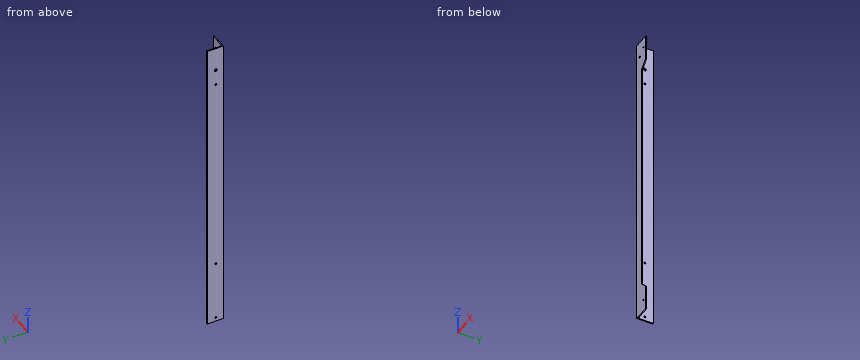
Autodesk Inventor part; units mm, degrees
ref_plane "YZ Plane" through (0, 0, 0) normal (1, 0, 0) x (0, 1, 0)
ref_plane "XZ Plane" through (0, 0, 0) normal (0, 1, 0) x (-1, 0, 0)
ref_plane "XY Plane" through (0, 0, 0) normal (0, 0, 1) x (1, 0, 0)
sketch "Sketch1" plane through (0, 0, 0) normal (0, 0, 1) x (1, 0, 0)
  line L0 (0, 0) -> (3.175, 0)
  line L1 (3.175, 0) -> (3.175, 50.8)
  line L2 (3.175, 50.8) -> (0, 50.8)
  line L3 (0, 50.8) -> (0, 0)
  line L4 (0, 0) -> (50.8, 0)
  line L5 (50.8, 0) -> (50.8, 3.175)
  line L6 (50.8, 3.175) -> (0, 3.175)
  line L7 (0, 3.175) -> (0, 0)
  dimension "d0" = 3.175
  dimension "d1" = 50.8
  dimension "d2" = 50.8
  dimension "d3" = 3.175
extrude "Extrusion1" add sketch "Sketch1" along normal blind 965.2
sketch "Sketch2" plane through (0, 0, 0) normal (-1, 0, 0) x (0, 0, 1)
  line L0 (0, 50.8) -> (0, 0)
  line L1 (0, 0) -> (965.2, 0)
  point P0 (12.7, 23.8125)
  point P1 (203.2, 23.8125)
  dimension "d6" = 23.8125
  dimension "d7" = 23.8125
  dimension "d8" = 12.7
  dimension "d9" = 203.2
hole "Hole1" at (0, 23.8125, 12.7) at (0, 23.8125, 203.2) direction (1, 0, 0) diameter 6.35 end through all
sketch "Sketch3" plane through (0, 0, 0) normal (-1, 0, 0) x (0, 0, 1)
  line L0 (0, 0) -> (965.2, 0)
  line L1 (0, 50.8) -> (0, 0)
  point P0 (889, 23.8125)
  dimension "d17" = 23.8125
  dimension "d26" = 889
hole "Hole2" at (0, 23.8125, 889) direction (1, 0, 0) diameter 9.525 end through all
sketch "Sketch4" plane through (0, 0, 0) normal (0, -1, 0) x (1, 0, 0)
  line L0 (0, 965.2) -> (50.8, 965.2)
  line L1 (0, 0) -> (0, 965.2)
  point P0 (17.4625, 914.4)
  dimension "d27" = 17.4625
  dimension "d28" = 50.8
hole "Hole3" at (17.4625, 0, 914.4) direction (0, 1, 0) diameter 6.35 end through all
fillet "Fillet1" radius 3.175 1 edges at (3.175, 3.175, 482.6)
sketch "Sketch6" plane through (0, 0, 0) normal (0, -1, 0) x (1, 0, 0)
  line L0 (0, 0) -> (50.8, 0)
  line L1 (50.8, 0) -> (50.8, 965.2)
  line L2 (0, 965.2) -> (50.8, 965.2)
  point P0 (38.1, 933.45)
  point P1 (38.1, 38.1)
  dimension "d49" = 38.1
  dimension "d50" = 12.7
  dimension "d51" = 31.75
  dimension "d52" = 12.7
hole "Hole5" at (38.1, 0, 933.45) at (38.1, 0, 38.1) direction (0, 1, 0) diameter 4.7625 end through all
sketch "Sketch8" plane through (0, 0, 0) normal (0, -1, 0) x (1, 0, 0)
  circle A0 centre (38.1, 933.45) radius 2.3813
  circle A1 centre (38.1, 38.1) radius 2.3813
  circle A2 centre (17.4625, 914.4) radius 3.175
  line L0 (0, 0) -> (50.8, 0)
  line L1 (50.8, 0) -> (50.8, 965.2)
  line L2 (0, 965.2) -> (50.8, 965.2)
  line L3 (0, 0) -> (0, 965.2)
  line L4 (50.8, 863.6) -> (28.575, 863.6)
  line L5 (28.575, 863.6) -> (28.575, 101.6)
  line L6 (28.575, 101.6) -> (50.8, 101.6)
  line L7 (50.8, 101.6) -> (50.8, 863.6)
  line L8 (28.575, 863.6) -> (50.8, 885.825)
  line L9 (50.8, 0) -> (50.8, 965.2)
  line L10 (28.575, 863.6) -> (60.0059, 863.6) construction
  line L11 (50.8, 885.825) -> (50.8, 863.6)
  line L12 (28.575, 101.6) -> (50.8, 79.375)
  line L13 (28.575, 101.6) -> (60.0059, 101.6) construction
  line L14 (50.8, 79.375) -> (50.8, 101.6)
  dimension "d60" = 22.225
  dimension "d61" = 101.6
  dimension "d62" = 101.6
  dimension "d63" = 45
  dimension "d64" = 45
extrude "Extrusion2" cut sketch "Sketch8" against normal blind 25.4 contours L12 L6 L1 | L6 L5 L4 L1 | L1 L4 L8
sketch "Sketch9" plane through (0, 0, 0) normal (-1, 0, 0) x (0, 0, 1)
  circle A0 centre (889, 23.8125) radius 4.7625
  circle A1 centre (12.7, 23.8125) radius 3.175
  circle A2 centre (203.2, 23.8125) radius 3.175
  line L0 (0, 50.8) -> (0, 0)
  line L1 (0, 0) -> (965.2, 0)
  line L2 (965.2, 50.8) -> (965.2, 0)
  line L3 (0, 50.8) -> (965.2, 50.8)
  point P0 (838.2, 23.8125)
  dimension "d67" = 23.8125
  dimension "d68" = 127
hole "Hole6" at (0, 23.8125, 838.2) direction (1, 0, 0) diameter 6.35 end through all
properties part number "rail support 2x2 angle" material "Aluminum 6061"
Check sheet for the modelled part. Datum: model origin and axes. Units: mm. Give positions to 0.01 mm unless a question says otherwise; leave off trailing zeros. Write each loop counter-clockwise with the first axis right and the second up, starting at its lowest first coordinate (ties: lowest second). Pieces come first, ordered by that corner, then holes. Notation, with made-up numbers: (20.25, 66) -> (66.25, 66) arc R33 ccw to (66.25, 101) -> close; hole circle Ø8 at (-32.5, -25). An arc over 180 degrees is marked (long way). One line per item, written item: value. Start each with the question number.
Item 1: Section check A-A on z = 65. Record the cut outline in (x, y) (3 decimals).
Item 2: Section check B-B on z = 748. Record the cut outline in (x, y) (3 decimals).
Item 3: Gauge pin test, flat ends, axial feed: pin 1 (12 mm diameter, centred on y = 14, z = 499.5, fed in from +X) (3 decimals); pin 2 (5.5 mm diameter, centred on x = 17.46, z = 914.4, fed in from -Y); pin 3 (3.5 mm diameter, centred on y = 2.5, z = 460.5, fed in from +X) (3 decimals); pin 4 (12 mm diameter, centred on x = 32.5, z = 585, fed in from +Y) (3 decimals). Record the tip position at first contact, or that the pin passes through.
Item 4: Material ranges on probe 1 along Y at (x, z) = (1.8, 203.2); probe 2 along Y at (x, z) = (1, 889) (3 decimals); probe 3 along X at (y, z) = (1, 933), recorded low to high. Write a range as from..to.
Item 5: Section check C-C on y = 39.5. Record the cut outline in (x, z) (3 decimals).
Results list:
1. outline: (0, 0) -> (50.8, 0) -> (50.8, 3.175) -> (6.35, 3.175) arc R3.175 cw to (3.175, 6.35) -> (3.175, 50.8) -> (0, 50.8) -> close
2. outline: (0, 0) -> (28.575, 0) -> (28.575, 3.175) -> (6.35, 3.175) arc R3.175 cw to (3.175, 6.35) -> (3.175, 50.8) -> (0, 50.8) -> close
3. pin 1: x = 3.175
3. pin 2: through
3. pin 3: x = 28.575
3. pin 4: y = 3.175
4. probe 1: 0..20.64, 26.99..50.8
4. probe 2: 0..19.05, 28.575..50.8
4. probe 3: 0..35.76, 40.44..50.8
5. outline: (0, 0) -> (3.175, 0) -> (3.175, 965.2) -> (0, 965.2) -> close
